from build123d import *

# Parameters (mm, degrees)
F0_R     = 10
F0_R_2   = 2.125
F1_DEPTH = 70
F2_W     = 23.7841829658
F2_H     = 12
F3_DEPTH = 50


with BuildPart() as f1:
    # F0 (on Front) → F1 (new body)
    with BuildSketch(Plane.XZ):
        with BuildLine():
            Line((60, 29.1429199278), (-60, 29.1429199278))
            Line((-60, 29.1429199278), (-75.0524420565, 40.3041392565))
            Line((-75.0524420565, 40.3041392565), (-93.0163642764, 40.3041392565))
            Line((-93.0163642764, 40.3041392565), (-73.4979985282, 20.4398736871))
            add(Edge.make_bspline(
                [(-77.6378661394, 0), (-78.1194158464, 4.7639785375), (-78.9848755826, 13.3259848022), (-75.1840223047, 18.2538969131), (-73.4979985282, 20.4398736871)],
                knots=[0, 0, 0, 0, 0.5564091394, 1, 1, 1, 1], degree=3))
            add(Edge.make_bspline(
                [(-16.6683998403, -29.1429199278), (-21.7410225995, -22.9682576809), (-32.5546179399, -10.6737549318), (-71.809926995, -17.7841787732), (-75.4187412252, -5.6402197394), (-77.6378661394, 0)],
                knots=[0, 0, 0, 0, 0.3300992596, 0.7296032213, 1, 1, 1, 1], degree=3))
            Line((-16.6683998403, -29.1429199278), (60, -29.1429199278))
            Line((60, -29.1429199278), (60, 29.1429199278))
        make_face()
        with Locations((-58.7333962321, 0)):
            Circle(F0_R, mode=Mode.SUBTRACT)
        with Locations((-79.928971827, 34.9695757031)):
            Circle(F0_R_2, mode=Mode.SUBTRACT)
        Polygon((321, 29.1429199278), (60, 29.1429199278), (60, -29.1429199278), align=None)
    extrude(amount=F1_DEPTH)

    # F2 (on Top) → F3 (cut, symmetric)
    with BuildSketch(Plane.XY):
        Polygon((-120.2781274915, 0), (-120.2781274915, -25), (-23.9695869386, -25), (-23.9695869386, 0), (-60, 0), align=None)
        Polygon((-23.9695869386, -45), (-122.6608380675, -45), (-122.6608380675, -72.7143883705), (-24.00202282, -72.7143883705), align=None)
        with Locations((-83.2946263254, -35)):
            Rectangle(F2_W, F2_H)
    extrude(amount=F3_DEPTH, both=True, mode=Mode.SUBTRACT)


solid = f1.part
For this review, take the finished solid that the model builds, in its own axes (mm). A direction names the side the tool comes from. Round coordinates to 2 decimals unless told otherwise and drop trailing zeros. Loops run counter-clockwise (first coordinate to the right, second up) from the corner with the lowest first, then second, coordinate; pieces in that order, holes last. Notation, with made-up numbers: (-9, 21.25) - (41, 21.25) arc R18 cw to (41, 52.25) - close; hole circle Ø8 at (-34, 64.25). An arc over 180 degrees is marked (long way). Use one line per item in the form item = value.
1) Mouldability with a two-part tool opening along X and no side actions: class faces 1 (the face through (-68.724, -34.86, 0.44)), 2 (the face through (-83.39, -26.97, 30.51)), 3 (the face through (133, -35, 29.143)) as pulls with the +X half, pulls with the -X half, needs draft (parallel to the pull), parting line crosses it, or undercut.
Solutions:
face_1 = undercut
face_2 = pulls with the -X half
face_3 = needs draft
2) We need section B-B on x = 118. Write out the cut boundary in (y, z), then the cut area to 3 significant figures.
Solutions:
outline = (-70, -16.19) - (0, -16.19) - (0, 29.14) - (-70, 29.14) - close
area = 3,170 mm2
3) We need section A-A on x = 167. Write out the cut boundary in (y, z), then the cut area to 3 significant figures.
Solutions:
outline = (-70, -5.25) - (0, -5.25) - (0, 29.14) - (-70, 29.14) - close
area = 2,410 mm2
4) Wall thickness on probe 1 along Z at (x, y) = (25, -20); probe 2 along Z at (x, y) = (234, -30.5); probe 3 along Z at (x, y) = (-56.5, -27): over which ranges is each line inside the solid? List them lowest first.
Solutions:
probe_1 = -29.14 to 29.14
probe_2 = 9.71 to 29.14
probe_3 = -14.33 to -9.75, 9.75 to 29.14
5) Clearance check with flat-ended pins moving along their axes: P1, Ø21, axis at x = 98, y = -49, coming from the +Z side; P2, Ø2.5, axis at x = -79.93, z = 34.97, coming from the -Y side; P3, Ø24, axis at x = -83, z = 17, coming from the +Y side; P4, Ø1.5, axis at y = -9.5, z = -15.5, coming from the -X side. State where each tip first meets the part, or that it passes through.
Solutions:
P1 = 29.14
P2 = through
P3 = -25
P4 = -23.97
6) Tool access review of faces 4 (the face through (-51, -25, 9)), 5 (the face through (-74, -29, 19)), 6 (the face through (-83.39, -42.97, 30.51)): name each direction out of +Z, -Z, +X, -X, +Y, -Y from which nothing blocks a thin tool from reaching the whole face with its end or side.
Solutions:
face_4 = +Z, -Z, -X, +Y
face_5 = +Z, -Z, -X
face_6 = -X, +Y, -Y
